```python
from build123d import *

# Parameters (mm, degrees)
SKETCH1_R             = 10
BOSS_EXTRUDE1_DEPTH   = 3
BOSS_EXTRUDE2_DEPTH   = 10
BOSS_EXTRUDE2_2_DEPTH = 10
BOSS_EXTRUDE3_DEPTH   = 3
SKETCH6_W             = 3
SKETCH6_H             = 253
BOSS_EXTRUDE4_DEPTH   = 159
BOSS_EXTRUDE6_DEPTH   = 10
SKETCH9_R             = 1.735
CUT_EXTRUDE3_DEPTH    = 10
BOSS_EXTRUDE7_DEPTH   = 80.27650967
CUT_EXTRUDE6_DEPTH    = 143
SKETCH14_W            = 253
SKETCH14_H            = 35
CUT_EXTRUDE7_DEPTH    = 143
CUT_EXTRUDE8_DEPTH    = 143
SKETCH17_R            = 2.5
CUT_EXTRUDE9_DEPTH    = 143
SKETCH18_W            = 12.581611653
SKETCH18_H            = 132.027792725
CUT_EXTRUDE10_DEPTH   = 143
SKETCH29_W            = 88.113599476
SKETCH29_H            = 135.236918358
CUT_EXTRUDE19_DEPTH   = 150


with BuildPart() as part:
    # Sketch1 → Boss-Extrude1 (new body)
    with BuildSketch(Plane(origin=(0, 0, 0), x_dir=(0, 0, -1), z_dir=(1, 0, 0))):
        with BuildLine():
            Line((-77.887006237, -82.154885655), (77.912993763, -82.154885655))
            Line((77.912993763, -82.154885655), (77.912993763, -78.154885655))
            ThreePointArc((77.912993763, -78.154885655), (86.412993763, -69.654885655), (94.912993763, -78.154885655))
            Line((94.912993763, -78.154885655), (94.912993763, -82.154885655))
            Line((94.912993763, -82.154885655), (125.012993763, -82.154885655))
            Line((125.012993763, -82.154885655), (125.012993763, 51.845114345))
            Line((125.012993763, 51.845114345), (-124.987006237, 51.845114345))
            Line((-124.987006237, 51.845114345), (-124.987006237, -82.154885655))
            Line((-124.987006237, -82.154885655), (-94.887006237, -82.154885655))
            Line((-94.887006237, -82.154885655), (-94.887006237, -78.154885655))
            ThreePointArc((-94.887006237, -78.154885655), (-86.387006237, -69.654885655), (-77.887006237, -78.154885655))
            Line((-77.887006237, -78.154885655), (-77.887006237, -82.154885655))
        make_face()
        with Locations((-101.987006237, -28.654885655)):
            Circle(SKETCH1_R, mode=Mode.SUBTRACT)
        with Locations(Location((102.012993763, -28.654885655, 0), (0, 0, 180))):
            Circle(SKETCH1_R, mode=Mode.SUBTRACT)
    extrude(amount=-BOSS_EXTRUDE1_DEPTH)

    # Sketch5 → Boss-Extrude3 (add)
    with BuildSketch(Plane(origin=(0, 0, 0), x_dir=(0, 0, -1), z_dir=(1, 0, 0))):
        with BuildLine():
            Line((-124.987006237, 76.845114345), (-124.987006237, 51.845114345))
            Line((-124.987006237, 51.845114345), (125.012993763, 51.845114345))
            Line((125.012993763, 51.845114345), (125.012993763, -82.154885655))
            Line((125.012993763, -82.154885655), (128.012993763, -82.154885655))
            Line((128.012993763, -82.154885655), (128.012993763, 56.845114345))
            ThreePointArc((128.012993763, 56.845114345), (122.155129387, 70.987249969), (108.012993763, 76.845114345))
            Line((108.012993763, 76.845114345), (-124.987006237, 76.845114345))
        make_face()
    extrude(amount=-BOSS_EXTRUDE3_DEPTH)



with BuildPart() as body_2:
    # Sketch2 → Boss-Extrude2 (new body)
    with BuildSketch(Plane.ZY.offset(3)):
        with BuildLine():
            Line((-75.012993763, 59.845114345), (-69.012993763, 59.845114345))
            ThreePointArc((-69.012993763, 59.845114345), (-68.305886982, 59.552221126), (-68.012993763, 58.845114345))
            Line((-68.012993763, 58.845114345), (-68.012993763, 54.845114345))
            ThreePointArc((-68.012993763, 54.845114345), (-68.305886982, 54.138007564), (-69.012993763, 53.845114345))
            Line((-69.012993763, 53.845114345), (-75.012993763, 53.845114345))
            ThreePointArc((-75.012993763, 53.845114345), (-75.720100544, 54.138007564), (-76.012993763, 54.845114345))
            Line((-76.012993763, 54.845114345), (-76.012993763, 58.845114345))
            ThreePointArc((-76.012993763, 58.845114345), (-75.720100544, 59.552221126), (-75.012993763, 59.845114345))
        make_face()
    extrude(amount=BOSS_EXTRUDE2_DEPTH)


with BuildPart() as body_3:
    # Sketch2 → Boss-Extrude2 2 (new body)
    with BuildSketch(Plane.ZY.offset(3)):
        with BuildLine():
            Line((67.987006237, 58.845114345), (67.987006237, 54.845114345))
            ThreePointArc((67.987006237, 54.845114345), (68.279899456, 54.138007564), (68.987006237, 53.845114345))
            Line((68.987006237, 53.845114345), (74.987006237, 53.845114345))
            ThreePointArc((74.987006237, 53.845114345), (75.694113018, 54.138007564), (75.987006237, 54.845114345))
            Line((75.987006237, 54.845114345), (75.987006237, 58.845114345))
            ThreePointArc((75.987006237, 58.845114345), (75.694113018, 59.552221126), (74.987006237, 59.845114345))
            Line((74.987006237, 59.845114345), (68.987006237, 59.845114345))
            ThreePointArc((68.987006237, 59.845114345), (68.279899456, 59.552221126), (67.987006237, 58.845114345))
        make_face()
    extrude(amount=BOSS_EXTRUDE2_2_DEPTH)


with BuildPart() as body_4:
    # Sketch6 → Boss-Extrude4 (new body)
    with BuildSketch(Plane(origin=(0, 76.845114345, 0), x_dir=(1, 0, 0), z_dir=(0, 1, 0))):
        with Locations((-84.77650967, 1.512993763)):
            Rectangle(SKETCH6_W, SKETCH6_H)
    extrude(amount=-BOSS_EXTRUDE4_DEPTH)

    # Sketch8 → Boss-Extrude6 (add)
    with BuildSketch(Plane.ZY.offset(83.27650967)):
        with BuildLine():
            Line((-75.012993763, 59.845114345), (-69.012993763, 59.845114345))
            ThreePointArc((-69.012993763, 59.845114345), (-68.305886982, 59.552221126), (-68.012993763, 58.845114345))
            Line((-68.012993763, 58.845114345), (-68.012993763, 54.845114345))
            ThreePointArc((-68.012993763, 54.845114345), (-68.305886982, 54.138007564), (-69.012993763, 53.845114345))
            Line((-69.012993763, 53.845114345), (-75.012993763, 53.845114345))
            ThreePointArc((-75.012993763, 53.845114345), (-75.720100544, 54.138007564), (-76.012993763, 54.845114345))
            Line((-76.012993763, 54.845114345), (-76.012993763, 58.845114345))
            ThreePointArc((-76.012993763, 58.845114345), (-75.720100544, 59.552221126), (-75.012993763, 59.845114345))
        make_face()
        with BuildLine():
            Line((68.987006237, 59.845114345), (74.987006237, 59.845114345))
            ThreePointArc((74.987006237, 59.845114345), (75.694113018, 59.552221126), (75.987006237, 58.845114345))
            Line((75.987006237, 58.845114345), (75.987006237, 54.845114345))
            ThreePointArc((75.987006237, 54.845114345), (75.694113018, 54.138007564), (74.987006237, 53.845114345))
            Line((74.987006237, 53.845114345), (68.987006237, 53.845114345))
            ThreePointArc((68.987006237, 53.845114345), (68.279899456, 54.138007564), (67.987006237, 54.845114345))
            Line((67.987006237, 54.845114345), (67.987006237, 58.845114345))
            ThreePointArc((67.987006237, 58.845114345), (68.279899456, 59.552221126), (68.987006237, 59.845114345))
        make_face()
    extrude(amount=-BOSS_EXTRUDE6_DEPTH)


with BuildPart() as cut_extrude3_tool:
    # Sketch9 → Cut-Extrude3 (new body)
    with BuildSketch(Plane(origin=(0, 59.845114345, 0), x_dir=(1, 0, 0), z_dir=(0, 1, 0))):
        with Locations(Location((-77.63650967, -71.987006237, 0), (0, 0, 270))):
            Circle(SKETCH9_R)
        with Locations(Location((-77.63650967, 72.012993763, 0), (0, 0, 270))):
            Circle(SKETCH9_R)
        with Locations(Location((-8.64, -71.987006237, 0), (0, 0, 270))):
            Circle(SKETCH9_R)
        with Locations(Location((-8.64, 72.012993763, 0), (0, 0, 270))):
            Circle(SKETCH9_R)
    extrude(amount=-CUT_EXTRUDE3_DEPTH)


with BuildPart() as body_2_1:
    add(body_2.part)

    # Cut-Extrude3: cut by cut_extrude3_tool
    add(cut_extrude3_tool.part, mode=Mode.SUBTRACT)


with BuildPart() as body_3_1:
    add(body_3.part)

    # Cut-Extrude3: cut by cut_extrude3_tool
    add(cut_extrude3_tool.part, mode=Mode.SUBTRACT)


with BuildPart() as body_4_1:
    add(body_4.part)

    # Cut-Extrude3: cut by cut_extrude3_tool
    add(cut_extrude3_tool.part, mode=Mode.SUBTRACT)


with BuildPart() as part_1:
    add(part.part)

    add(body_4_1.part)  # Boss-Extrude7 merges body 4
    # Sketch11 → Boss-Extrude7 (add)
    with BuildSketch(Plane.ZY.offset(3)):
        with BuildLine():
            Line((124.987006237, 73.845114345), (124.987006237, 76.845114345))
            Line((124.987006237, 76.845114345), (-108.012993763, 76.845114345))
            ThreePointArc((-108.012993763, 76.845114345), (-122.155129387, 70.987249969), (-128.012993763, 56.845114345))
            Line((-128.012993763, 56.845114345), (-128.012993763, -82.154885655))
            Line((-128.012993763, -82.154885655), (-125.012993763, -82.154885655))
            Line((-125.012993763, -82.154885655), (-125.012993763, 56.845114345))
            ThreePointArc((-125.012993763, 56.845114345), (-120.033809043, 68.865929625), (-108.012993763, 73.845114345))
            Line((-108.012993763, 73.845114345), (124.987006237, 73.845114345))
        make_face()
    extrude(amount=BOSS_EXTRUDE7_DEPTH)

    # Sketch13 → Cut-Extrude6 (cut)
    with BuildSketch(Plane(origin=(0, 0, 0), x_dir=(0, 0, -1), z_dir=(1, 0, 0))):
        with BuildLine():
            Line((-111.987006237, -28.654885655), (-111.987006237, -82.154885655))
            Line((-111.987006237, -82.154885655), (-77.887006237, -82.154885655))
            Line((-77.887006237, -82.154885655), (-77.887006237, -78.154885655))
            ThreePointArc((-77.887006237, -78.154885655), (-80.376598597, -72.144478015), (-86.387006237, -69.654885655))
            Line((-86.387006237, -69.654885655), (-86.387006237, -28.654885655))
            ThreePointArc((-86.387006237, -28.654885655), (-89.315938425, -21.583817843), (-96.387006237, -18.654885655))
            Line((-96.387006237, -18.654885655), (-101.987006237, -18.654885655))
            ThreePointArc((-101.987006237, -18.654885655), (-109.058074049, -21.583817843), (-111.987006237, -28.654885655))
        make_face()
        with BuildLine():
            Line((112.012993763, -82.154885655), (112.012993763, -28.654885655))
            ThreePointArc((112.012993763, -28.654885655), (109.084061575, -21.583817843), (102.012993763, -18.654885655))
            Line((102.012993763, -18.654885655), (96.412993763, -18.654885655))
            ThreePointArc((96.412993763, -18.654885655), (89.341925951, -21.583817843), (86.412993763, -28.654885655))
            Line((86.412993763, -28.654885655), (86.412993763, -69.654885655))
            ThreePointArc((86.412993763, -69.654885655), (80.402586123, -72.144478015), (77.912993763, -78.154885655))
            Line((77.912993763, -78.154885655), (77.912993763, -82.154885655))
            Line((77.912993763, -82.154885655), (112.012993763, -82.154885655))
        make_face()
    extrude(amount=-CUT_EXTRUDE6_DEPTH, mode=Mode.SUBTRACT)

    # Sketch14 → Cut-Extrude7 (cut)
    with BuildSketch(Plane(origin=(0, 0, 0), x_dir=(0, 0, -1), z_dir=(1, 0, 0))):
        with Locations((1.512993763, -64.654885655)):
            Rectangle(SKETCH14_W, SKETCH14_H)
    extrude(amount=-CUT_EXTRUDE7_DEPTH, mode=Mode.SUBTRACT)

    # Sketch15 → Cut-Extrude8 (cut)
    with BuildSketch(Plane(origin=(0, 0, 0), x_dir=(0, 0, -1), z_dir=(1, 0, 0))):
        with BuildLine():
            Line((108.012993763, 76.845114345), (128.012993763, 76.845114345))
            Line((128.012993763, 76.845114345), (128.012993763, 56.845114345))
            ThreePointArc((128.012993763, 56.845114345), (122.155129387, 70.987249969), (108.012993763, 76.845114345))
        make_face()
    extrude(amount=-CUT_EXTRUDE8_DEPTH, mode=Mode.SUBTRACT)

    # Sketch17 → Cut-Extrude9 (cut)
    with BuildSketch(Plane(origin=(0, 76.845114345, 0), x_dir=(1, 0, 0), z_dir=(0, 1, 0))):
        with Locations(Location((-43.138761, -96.337006347, 0), (0, 0, 270))):
            Circle(SKETCH17_R)
    extrude(amount=-CUT_EXTRUDE9_DEPTH, mode=Mode.SUBTRACT)

    # Sketch18 → Cut-Extrude10 (cut)
    with BuildSketch(Plane(origin=(0, 0, 0), x_dir=(0, 0, -1), z_dir=(1, 0, 0))):
        with Locations((-126.277812064, 15.020453299)):
            Rectangle(SKETCH18_W, SKETCH18_H)
    extrude(amount=-CUT_EXTRUDE10_DEPTH, mode=Mode.SUBTRACT)


with BuildPart() as cut_extrude19_tool:
    # Sketch29 → Cut-Extrude19 (new, symmetric)
    with BuildSketch(Plane.XY):
        with Locations((-28.779229361, 13.195273746)):
            Rectangle(SKETCH29_W, SKETCH29_H)
    extrude(amount=CUT_EXTRUDE19_DEPTH, both=True)


with BuildPart() as part_2:
    add(part_1.part)

    # Cut-Extrude19: cut by cut_extrude19_tool
    add(cut_extrude19_tool.part, mode=Mode.SUBTRACT)


with BuildPart() as body_2_2:
    add(body_2_1.part)

    # Cut-Extrude19: cut by cut_extrude19_tool
    add(cut_extrude19_tool.part, mode=Mode.SUBTRACT)


with BuildPart() as body_3_2:
    add(body_3_1.part)

    # Cut-Extrude19: cut by cut_extrude19_tool
    add(cut_extrude19_tool.part, mode=Mode.SUBTRACT)


solid = part_2.part
```
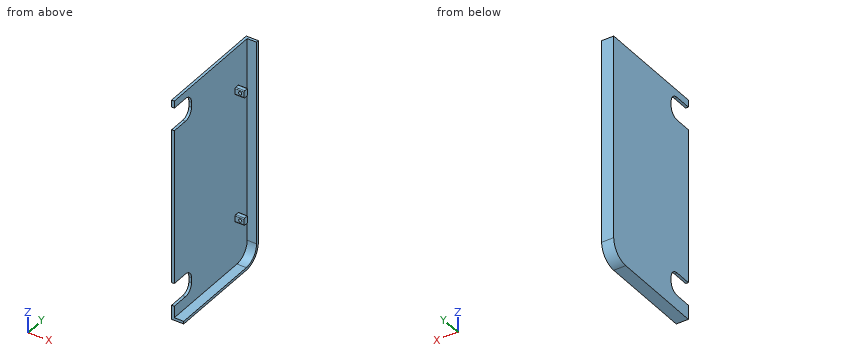
Input: part model. Units: mm. Frame: model coordinates. Give positions to 0.01 mm unless a question says otherwise; leave off trailing zeros. Order: outer loops, then holes, each group sorted by start corner. A loop starts at its lowest first (then second) coordinate and runs counter-clockwise, first axis right, second up. Notation, with made-up numbers: (73, 74) -> (82, 74) arc R27 ccw to (82, 92) -> close; hole circle Ø3 at (10.25, 73.5). An arc over 180 degrees is marked (long way). Write each question's results on one line, items separated by ' | '. Start each with the question number.
Item 1: Cut plane B-B on z = 37. Return the cut outline in (x, y).
Item 2: Contact query for flat-ended pins moving along their axis: P1, Ø5, axis at y = 58.5, z = 73, coming from the +X side; P2, Ø1.5, axis at y = -17, z = 71.5, coming from the +X side; P3, Ø8, axis at x = -75.5, y = 6, coming from the +Z side. Output: stop coordinate, or through.
Item 3: Cut plane A-A on y = 34. Return the cut outline in (x, z), then the cut area to 3 significant figures.
Item 4: Line query: line 1 (Z direction, x = -82, y = 56); line 2 (Z direction, x = -85.25, y = -23); line 3 (Y direction, x = -74.5, z = -70.5). Output: solid intervals per line, ascending.
Established:
1) outline: (-86.28, -47.15) -> (-83.28, -47.15) -> (-83.28, 73.85) -> (-72.84, 73.85) -> (-72.84, 76.85) -> (-86.28, 76.85) -> close
2) P1: x = -73.28 | P2: x = -83.28 | P3: z = -125.01
3) outline: (-86.28, -128.01) -> (-72.84, -128.01) -> (-72.84, -125.01) -> (-83.28, -125.01) -> (-83.28, 119.99) -> (-86.28, 119.99) -> close | area: 775 mm^2
4) line 1: -128.01 to -125.01, -76.01 to -68.01, 67.99 to 75.99 | line 2: -128.01 to -110.26, -88.17 to 88.14, 110.23 to 119.99 | line 3: 53.85 to 59.85, 73.85 to 76.85
